from build123d import *

# Parameters (mm, degrees)
BOSS_EXTRUDE1_DEPTH = 120
BOSS_EXTRUDE2_DEPTH = 10
SKETCH3_R           = 9.25
SKETCH3_R_2         = 1.5
CUT_EXTRUDE1_DEPTH  = 10
FILLET1_R           = 10
SKETCH4_R           = 5
CUT_EXTRUDE2_DEPTH  = 20
FILLET2_R           = 10
FILLET4_R           = 10
FILLET6_R           = 10
SKETCH5_R           = 2.5
CUT_EXTRUDE3_DEPTH  = 5


with BuildPart() as part:
    # Sketch1 → Boss-Extrude1 (new body)
    with BuildSketch(Plane.XY):
        with BuildLine():
            Line((0, 0), (-70, 0))
            ThreePointArc((-70, 0), (-72.966131028, 40), (-70, 80))
            Line((-70, 80), (-70, 90))
            Line((-70, 90), (-170, 90))
            Line((-170, 90), (-170, 80))
            Line((-170, 80), (-80, 80))
            Line((-80, 80), (-80, -10))
            Line((-80, -10), (0, -10))
            Line((0, -10), (0, 0))
        make_face()
    extrude(amount=BOSS_EXTRUDE1_DEPTH)

    # Sketch2 → Boss-Extrude2 (add)
    with BuildSketch(Plane.ZY.offset(170)):
        with BuildLine():
            Line((0, 80), (0, 77.669175799))
            ThreePointArc((0, 77.669175799), (60, 17.669175799), (120, 77.669175799))
            Line((120, 77.669175799), (120, 90))
            Line((120, 90), (0, 90))
            Line((0, 90), (0, 80))
        make_face()
    extrude(amount=BOSS_EXTRUDE2_DEPTH)

    # Sketch3 → Cut-Extrude1 (cut)
    with BuildSketch(Plane.ZY.offset(180)):
        with Locations((60, 53.8345879)):
            Circle(SKETCH3_R)
        with Locations((48, 46.906384669)):
            Circle(SKETCH3_R_2)
        with Locations((60, 67.69099436)):
            Circle(SKETCH3_R_2)
        with Locations((72, 46.906384669)):
            Circle(SKETCH3_R_2)
    extrude(amount=-CUT_EXTRUDE1_DEPTH, mode=Mode.SUBTRACT)

    # Fillet1
    fillet1_edges = [part.edges().sort_by_distance(p)[0] for p in [
        (0, -5, 0),
        (0, -5, 120),
    ]]
    fillet(fillet1_edges, radius=FILLET1_R)

    # Sketch4 → Cut-Extrude2 (cut)
    with BuildSketch(Plane(origin=(0, 0, 0), x_dir=(1, 0, 0), z_dir=(0, 1, 0))):
        with Locations(Location((-35, -25, 0), (0, 0, 180))):
            Circle(SKETCH4_R)
        with Locations(Location((-35, -95, 0), (0, 0, 180))):
            Circle(SKETCH4_R)
    extrude(amount=-CUT_EXTRUDE2_DEPTH, mode=Mode.SUBTRACT)

    # Fillet2
    fillet2_edges = [part.edges().sort_by_distance(p)[0] for p in [
        (-70, 90, 60),
    ]]
    fillet(fillet2_edges, radius=FILLET2_R - 0.0001)  # a hair under: the kernel refuses the full size

    # Fillet4
    fillet4_edges = [part.edges().sort_by_distance(p)[0] for p in [
        (-80, 80, 60),
    ]]
    fillet(fillet4_edges, radius=FILLET4_R)

    # Fillet6
    fillet6_edges = [part.edges().sort_by_distance(p)[0] for p in [
        (-180, 90, 60),
    ]]
    fillet(fillet6_edges, radius=FILLET6_R)

    # Sketch5 → Cut-Extrude3 (cut)
    with BuildSketch(Plane.ZY.offset(180)):
        with Locations((72, 46.906384669)):
            Circle(SKETCH5_R)
        with Locations((60, 67.69099436)):
            Circle(SKETCH5_R)
        with Locations((48, 46.906384669)):
            Circle(SKETCH5_R)
    extrude(amount=-CUT_EXTRUDE3_DEPTH, mode=Mode.SUBTRACT)


solid = part.part
Geometry: final body of the model. Coordinates: model frame, mm. A direction names the side the tool comes from. Round coordinates to 2 decimals unless told otherwise and drop trailing zeros. Order: outer loops, then holes, each group sorted by start corner. A loop starts at its lowest first (then second) coordinate and runs counter-clockwise, first axis right, second up. Notation, with made-up numbers: (39, -26.75) -> (81, -26.75) arc R17 ccw to (81, -7.75) -> close; hole circle Ø9 at (-17, -21). An arc over 180 degrees is marked (long way). Put each result on its own line as item: value. Start each with the question number.
Q1. Pull-direction query (Y, two-part tool) for faces 1 (the cylindrical face through (-3.01, -4.93, 117.15)), 2 (the flat face through (-175, 45, 48)), 3 (the cylindrical face through (-82.85, 76.99, 60.84)); classes: +Y half, -Y half, draft (parallel to the pull), parting line (faces both ways), or undercut.
Q2. Section D-D on y = 25. Return the cut outline in (x, z), and give its area (3 significant figures).
Q3. Section A-A on x = -35. Return the cut outline in (y, z), and give its area (3 significant figures).
Q4. Line query: probe 1 along Z at (x, y) = (-35, -7.5); probe 2 along X at (y, z) = (42.5, 90); probe 3 along Y at (x, z) = (-177.5, 60). Output: solid intervals per line, ascending.
Q5. Section C-C on y = -2.5. Return the cut outline in (x, z).
Q6. Reachability of faces 4 (the cylindrical face through (-3.01, -4.93, 2.85)), 5 (the cylindrical face through (-177.54, 48.6, 70.16)), 6 (the flat face through (-80, 31, 59)), 7 (the flat face through (-35, 0, 59)) from +Z, -Z, +X, -X, +Y, -Y: full face, straight path, thin tool, end or side. Return the list, or none.
Q7. First-contact query: pin 1 (4 mm diameter, centred on x = -33, z = 29, fed in from +Y); pin 2 (24 mm diameter, centred on y = 53.83, z = 60, fed in from +X); pin 3 (4.5 mm diameter, centred on y = 46.91, z = 48, fed in from -X); pin 4 (13 mm diameter, centred on x = -35, z = 95, fed in from -Y). Flat tips, straight axial feed; report the tip coordinate or a pass-through.
Ans:
1. face 1: draft
1. face 2: undercut
1. face 3: -Y half
2. outline: (-180, 31.26) -> (-170, 31.26) -> (-170, 88.74) -> (-180, 88.74) -> close; (-80, 0) -> (-72.55, 0) -> (-72.55, 120) -> (-80, 120) -> close
2. area: 1,470 mm2
3. outline: (-10, 0) -> (0, 0) -> (0, 20) -> (-10, 20) -> close; (-10, 30) -> (0, 30) -> (0, 90) -> (-10, 90) -> close; (-10, 100) -> (0, 100) -> (0, 120) -> (-10, 120) -> close
3. area: 1,000 mm2
4. probe 1: z = 0 to 20, 30 to 90, 100 to 120
4. probe 2: x = -180 to -170, -80 to -72.95
4. probe 3: y = 17.67 to 44.58, 63.08 to 65.19, 70.19 to 86.61
5. outline: (-80, 0) -> (-10, 0) arc R10 ccw to (0, 10) -> (0, 110) arc R10 ccw to (-10, 120) -> (-80, 120) -> close; hole circle Ø10 at (-35, 25); hole circle Ø10 at (-35, 95)
6. face 4: -Z, +X, +Y, -Y
6. face 5: -X
6. face 6: +Z, -Z, -Y
6. face 7: +Z, -Z, +X, +Y
7. pin 1: stops at y = 0
7. pin 2: stops at x = -71.73
7. pin 3: stops at x = -175
7. pin 4: stops at y = -10
